Read the model definition and answer for the solid it produces. Units are mm, in the model's axes. Face numbers are marked on the shaded views. A direction names the side the tool comes from. Coordinates: 2 decimals unless noted, no trailing zeros. Loops run counter-clockwise (first coordinate to the right, second up) from the corner with the lowest first, then second, coordinate; pieces in that order, holes last. Notation, with made-up numbers: (-23.5, -40) -> (-16.5, -40) arc R16 ccw to (-16.5, -9) -> close; hole circle Ø5 at (-25, -20.5). An arc over 180 degrees is marked (long way). One line per question, with ' | ' between items. Start each with the question number.
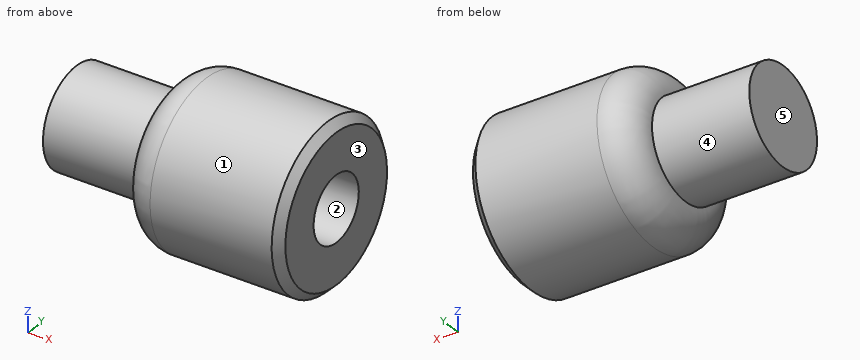
```python
from build123d import *

# Parameters (mm, degrees)
F2_SIZE = 0.5


with BuildPart() as f1:
    # F0 (on Front) → F1 (revolve)
    with BuildSketch(Plane.XZ):
        with BuildLine():
            Line((10, 5), (2, 5))
            ThreePointArc((2, 5), (0.585786, 4.414214), (0, 3))
            Line((0, 3), (-6, 3))
            Line((-6, 3), (-6, 0))
            Line((-6, 0), (0, 0))
            Line((0, 0), (2, 0))
            ThreePointArc((2, 0), (2.87868, 2.12132), (5, 3))
            Line((5, 3), (5, 2))
            Line((5, 2), (10, 2))
            Line((10, 2), (10, 5))
        make_face()
    revolve(axis=Axis((6.397376, 0, 0), (1, 0, 0)))

    # F2
    f2_edges = [f1.edges().sort_by_distance(p)[0] for p in [
        (10, 0, -5),
    ]]
    chamfer(f2_edges, length=F2_SIZE)


solid = f1.part
```
(1) Section A-A on x = 9 is taken. Write down the section's boundary in (y, z).
(2) A tool of negligible diameter and unlimited length cuts with its end or side. For the marked faces 4 and 5, from which of +Z, -Z, +X, -X, +Y, -Y can it reach the whole face along a straight path? Write none if from no direction.
(3) Determine the mould class of the marked faces 1, 2 and 3 for opening direction Y: +Y half, -Y half, draft (parallel to the pull), parting line (faces both ways), or undercut.
(4) Each of these flat-tipped pins is pushed along its axis until it touches: pin 1 Ø2 at (x, z) = (0.5, 0) entering from -Y; pin 2 Ø6 at (x, z) = (8, -3.5) entering from -Y. Where does it stop, or does it pass through?
(5) Find the intervals of material crossed by probe 1 along X at (y, z) = (1, -2); probe 2 along Y at (x, z) = (8.15, 0), in increasing order. Write a range as from..to.
(6) Section B-B on x = 1.5 is taken. Write down the section's boundary in (y, z).
Working result:
1) outline: circle Ø10 at (0, 0); hole circle Ø4 at (0, 0)
2) face 4: -X | face 5: +Z, -Z, -X, +Y, -Y
3) face 1: parting line | face 2: undercut | face 3: draft
4) pin 1: stops at y = -4.94 | pin 2: stops at y = -4.97
5) probe 1: x = -6..3, 5..10 | probe 2: y = -5..-2, 2..5
6) outline: circle Ø9.87 at (0, 0)
